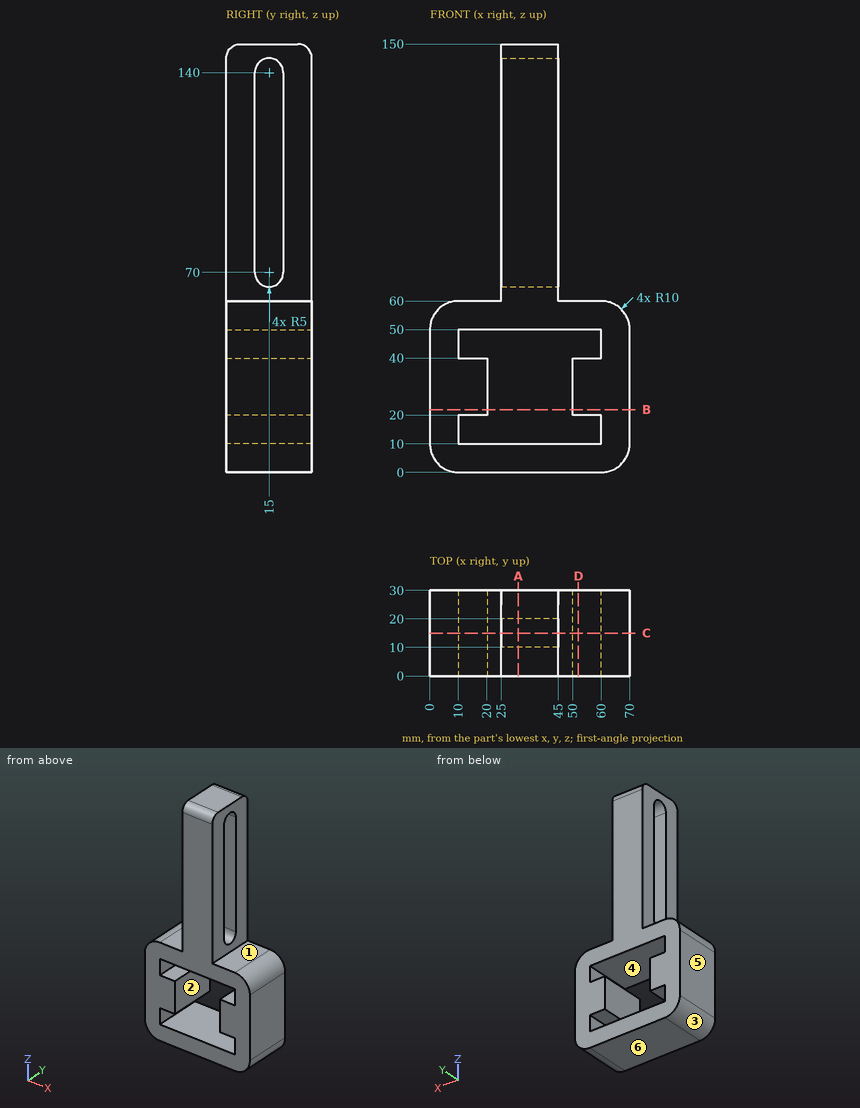
Verification items for this drawing (mm, ordinates from the low corner). A direction names the side the tool comes from. Give positions to 0.01 mm unless a question says otherwise; leave off trailing zeros. Loops run counter-clockwise (first coordinate to the right, second up) from the corner with the lowest first, then second, coordinate; pieces in that order, holes last. Notation, with made-up numbers: M 20,16.25 L 67,16.25 A12 ccw 67,21.25 Z; hole C 49.5,21.5 d6. An arc over 180 degrees is marked long. Return JSON: item names as keys, results as strings. Group by question number.
1. Cross-section at C-C on y = 15. Record the boundary of the cut face in (x, z).
2. Mould release check, pull along X, two halves, no side actions. Record for the marked faces 4, 5 and 6: released by +X, released by -X, zero draft, split by the parting line, or undercut.
3. Thickness scan on L1, parallel to Z at x = 13.5, y = 19; L2, parallel to Z at x = 46.5, y = 14.25; L3, parallel to X at y = 22, z = 25. Record the ranges inside material, lowest first.
4. Cross-section at B-B on z = 22. Record the boundary of the cut face in (x, y), plus the area to 3 significant figures.
5. Tool access check on the marked faces 1, 2 and 3. Record the directions out of +Z, -Z, +X, -X, +Y, -Y that give a thin tool (end or side, any length) a straight path to the whole face; none if there is none.
6. Cross-section at D-D on x = 52. Record the boundary of the cut face in (y, z).
7. Cross-section at A-A on x = 31. Record the boundary of the cut face in (y, z).
8. Go/stop test with flat-tipped pins: pin 1 (16.5 mm diameter, centred on x = 50.5, y = 15, fed in from +Z); pin 2 (9 mm diameter, centred on y = 19, z = 102.5, fed in from -X); pin 3 (12 mm diameter, centred on x = 17.5, y = 19.5, fed in from +Z); pin 4 (5 mm diameter, centred on x = 45.5, z = 19, fed in from -Y). Record where each tip stops, or that it passes through.
Return value:
{
 "1": {"outline": "M 0,10 A10 ccw 10,0 L 60,0 A10 ccw 70,10 L 70,50 A10 ccw 60,60 L 45,60 L 45,65 L 25,65 L 25,60 L 10,60 A10 ccw 0,50 Z; M 25,145 L 45,145 L 45,150 L 25,150 Z; hole M 10,10 L 60,10 L 60,20 L 50,20 L 50,40 L 60,40 L 60,50 L 10,50 L 10,40 L 20,40 L 20,20 L 10,20 Z"},
 "2": {"face 4": "undercut", "face 5": "released by -X", "face 6": "zero draft"},
 "3": {"L1": "0 to 10, 20 to 40, 50 to 60", "L2": "0 to 10, 50 to 60", "L3": "0 to 20, 50 to 70"},
 "4": {"outline": "M 0,0 L 20,0 L 20,30 L 0,30 Z; M 50,0 L 70,0 L 70,30 L 50,30 Z", "area": "1,200 mm^2"},
 "5": {"face 1": "+Z, +X, +Y, -Y", "face 2": "+Y, -Y", "face 3": "-Z, -X, +Y, -Y"},
 "6": {"outline": "M 0,0 L 30,0 L 30,10 L 0,10 Z; M 0,20 L 30,20 L 30,40 L 0,40 Z; M 0,50 L 30,50 L 30,60 L 0,60 Z"},
 "7": {"outline": "M 0,0 L 30,0 L 30,10 L 0,10 Z; M 0,50 L 30,50 L 30,145 A5 ccw 25,150 L 5,150 A5 ccw 0,145 Z; hole M 10,70 A5 ccw 20,70 L 20,140 A5 ccw 10,140 Z"},
 "8": {"pin 1": "z = 150", "pin 2": "x = 25", "pin 3": "z = 60", "pin 4": "through"}
}
